Autodesk Inventor part; units mm, degrees
ref_plane "YZ Plane" through (0, 0, 0) normal (1, 0, 0) x (0, 1, 0)
ref_plane "XZ Plane" through (0, 0, 0) normal (0, 1, 0) x (-1, 0, 0)
ref_plane "XY Plane" through (0, 0, 0) normal (0, 0, 1) x (1, 0, 0)
sketch "Sketch1" plane through (0, 0, 0) normal (0, 1, 0) x (-1, 0, 0)
  line L0 (0, 0) -> (0, 84.5) construction
  line L1 (0, 84.5) -> (-59.750523, 144.250523) construction
  line L2 (63.2, 0) -> (55, 0)
  line L3 (55, 0) -> (55, 61)
  line L4 (55, 61) -> (63.2, 61)
  line L5 (63.2, 61) -> (63.2, 0)
  line L6 (0, 0) -> (55, 0) construction
  line L7 (55, 61) -> (0, 61) construction
  line L8 (-20.85965, 183.141396) -> (22.273864, 140.007882)
  line L9 (22.273864, 140.007882) -> (28.072139, 145.806158)
  line L10 (28.072139, 145.806158) -> (-15.061374, 188.939672)
  line L11 (-15.061374, 188.939672) -> (-20.85965, 183.141396)
  line L12 (22.273864, 140.007882) -> (-16.617009, 101.117009) construction
  line L13 (-20.85965, 183.141396) -> (-59.750523, 144.250523) construction
  arc A0 (0, 61) -> (-16.617009, 101.117009) centre (-56.734019, 61) ccw
  line L14 (28.072139, 145.806158) -> (30.897031, 142.981266)
  line L15 (30.897031, 142.981266) -> (25.098755, 137.182991)
  line L16 (25.098755, 137.182991) -> (22.273864, 140.007882)
  line L17 (55, 61) -> (55, 64.995) construction
  line L18 (55, 64.995) -> (63.2, 64.995)
  line L19 (63.2, 64.995) -> (63.2, 61)
  line L20 (-15.061374, 188.939672) -> (-59.750523, 144.250523)
  line L21 (-15.061374, 188.939672) -> (30.897031, 142.981266)
  line L22 (30.897031, 142.981266) -> (-13.792118, 98.292118)
  line L23 (-13.792118, 98.292118) -> (-59.750523, 144.250523)
  line L24 (63.2, 64.995) -> (0, 64.995)
  line L25 (0, 64.995) -> (0, 0)
  line L26 (63.2, 0) -> (63.2, 64.995)
  line L27 (0, 0) -> (63.2, 0)
  line L28 (55, 61) -> (0, 61)
  line L29 (52.25, 64.995) -> (52.25, 61)
  line L30 (20.32932, 138.063339) -> (23.154212, 135.238447)
  line L31 (20.32932, 138.063339) -> (22.273864, 140.007882)
  dimension "d0" = 61
  dimension "d1" = 23.5
  dimension "d2" = 110
  dimension "d3" = 8.2
  dimension "d4" = 8.2
  dimension "d5" = 110
  dimension "d6" = 135
  dimension "d7" = 61
  dimension "d8" = 23.5
  dimension "d9" = 3.995
  dimension "d10" = 3.995
  dimension "d11" = 104.5
  dimension "d12" = 104.5
revolve "Revolution1" add sketch "Sketch1" angle 360 about axis through (0, 0, 84.5) along (0.7071068, 0, 0.7071068) contours L11 L10 L9 L8 | L8 L31 L30 L22 L23 L20 | L9 L14 L15 L16 | L16 L22 L30 L31
revolve "Revolution2" add sketch "Sketch1" angle 360 about axis through (0, 0, 0) along (0, 0, 1) contours L2 L3 L4 L5 | L27 L25 L28 L3 | L4 L28 L29 L24 L18 L19 | L28 L25 L24 L29
revolve "Revolution3" cut sketch "Sketch1" angle 360 about axis through (0, 0, 0) along (0, 0, 1) contours L27 L25 L28 L3 | L28 L25 L24 L29
revolve "Revolution4" cut sketch "Sketch1" angle 360 about axis through (0, 0, 84.5) along (0.7071068, 0, 0.7071068) contours L8 L31 L30 L22 L23 L20
sketch "Sketch2" plane through (0, 0, 64.995) normal (0, 0, 1) x (1, 0, 0)
  line L0 (47.089236, 42.152626) -> (47.089236, -42.152626)
  arc A0 (47.089236, 42.152626) -> (47.089236, -42.152626) centre (0, 0) ccw
  circle A1 centre (0, 0) radius 63.2
  circle A2 centre (0, 0) radius 52.25
  line L1 (47.079236, -42.163795) -> (47.079236, 42.163795)
  dimension "d13" = 104.5
  dimension "d14" = 126.4
  dimension "d15" = 0.01
revolve "Revolution5" add sketch "Sketch2" angle 45 about axis through (47.079236, -42.163795, 64.995) along (0, 1, 0) contours L1 A2 A0 | L1 A2
sketch "Sketch3" plane through (0, 0, 64.995) normal (0, 0, 1) x (1, 0, 0)
  circle A0 centre (0, 0) radius 52.25
  line L0 (47.089236, 42.152626) -> (47.089236, -42.152626)
  arc A1 (47.089236, 42.152626) -> (47.089236, -42.152626) centre (0, 0) ccw
  line L1 (53.089236, 110) -> (53.089236, -110)
  line L2 (-63.2, 0) -> (0, 0) construction
  point P0 (53.089236, 0)
  dimension "d17" = 6
  dimension "d18" = 220
revolve "Revolution6" cut sketch "Sketch3" angle 45 about axis through (53.089236, 110, 64.995) along (0, 1, 0) contours A0 L0 | L0 A0
equation "\"d0\" = t1"
equation "\"d1\" = z1"
equation "\"d2\" = dd1"
equation "\"d3\" = s1"
equation "\"d4\" = s1"
equation "\"d5\" = dd1"
equation "\"d7\" = t1"
equation "\"d8\" = z1"
equation "\"z1\" = 23.5"
equation "\"t1\" = 61"
equation "\"s1\" = 8.2"
equation "\"dd1\" = 110"
equation "\"X\" = 0.01"
equation "\"Y\" = 6"
properties part number "DIN 8063 Изгиб 45 градусов, тип W2 110" material "ПВХ, непластифицированный"
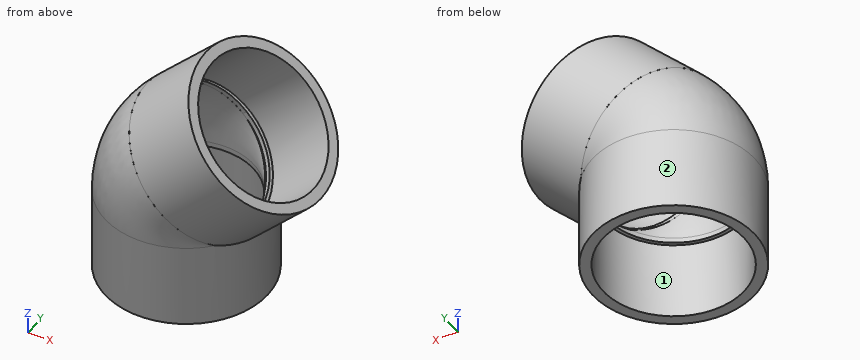
Input: part model. Units: mm. Frame: model coordinates. Face numbers are marked on the shaded views. Give positions to 0.01 mm unless a question says otherwise; leave off trailing zeros.
1. Draft query along X for the marked faces 1 and 2. Return one class per face: released by +X, released by -X, zero draft, split by the parting line, or undercut.
Computed:
face 1: undercut
face 2: split by the parting line
2. Cut plane A-A (z = 130). State how many separate pieces and enclosed holes the cut face has, and give its area (3 significant figures).
Computed:
separate pieces: 3
enclosed holes: 0
area: 2,700 mm2
3. Line query: probe 1 along X at (y, z) = (0, 24); probe 2 along X at (y, z) = (0, 63.3). Output: solid intervals per line, ascending.
Computed:
probe 1: x = -63.2 to -55, 55 to 63.2
probe 2: x = -63.2 to -52.25, 52.69 to 54.43, 56.58 to 68.18
4. Pin query (flat end, axial travel): pin 1 Ø1.5 at (x, z) = (3.5, 112.5) entering from +Y; pin 2 Ø10 at (x, y) = (-22.5, -12) entering from -Z; pin 3 Ø6 at (x, y) = (48, -16.5) entering from +Z. Return the tip coordinate at first contact, or that it passes through.
Computed:
pin 1: stops at y = 60.99
pin 2: stops at z = 130.32
pin 3: stops at z = 65.73
